```python
from build123d import *

# Parameters (mm, degrees)
F0_W         = 65
F0_H         = 45
F1_DEPTH     = 20
F2_T         = 5
F3_T1_DEPTH  = 19
F3_T3_DEPTH  = 63
F3_T5_DEPTH  = 43
F3_S9_W      = 1
F3_S9_H      = 1
F3_T10_DEPTH = 1
F3_S15_W     = 1
F3_S15_H     = 1
F3_T16_DEPTH = 1
F3_S21_W     = 1
F3_S21_H     = 1
F3_T22_DEPTH = 1
F3_S27_W     = 1
F3_S27_H     = 1
F3_T28_DEPTH = 1


# Not quite as in the source:
# - a fillet or chamfer that OpenCascade refuses, or shapes differently, is made with other operations: its cross-section is extruded or revolved along the edge and cut away or added


with BuildPart() as f1:
    # F0 (on Top) → F1 (new body)
    with BuildSketch(Plane.XY):
        Rectangle(F0_W, F0_H)
    extrude(amount=F1_DEPTH)

    # F2
    f2_openings = [f1.faces().sort_by_distance(p)[0] for p in [
        (0, 0, 20),
    ]]
    offset(amount=F2_T, openings=f2_openings, kind=Kind.INTERSECTION)

    # F3: fillet of radius 1 on 8 edges, made by hand

    # F3_s2 → F3_t1 (join)
    with BuildSketch(Plane.XY.offset(1)):
        with BuildLine():
            ThreePointArc((31.5, 22.5), (32.2071067812, 22.2071067812), (32.5, 21.5))
            Line((32.5, 21.5), (32.5, 22.5))
            Line((32.5, 22.5), (31.5, 22.5))
        make_face()
        with BuildLine():
            ThreePointArc((-31.5, 22.5), (-32.2071067812, 22.2071067812), (-32.5, 21.5))
            Line((-32.5, 21.5), (-32.5, 22.5))
            Line((-32.5, 22.5), (-31.5, 22.5))
        make_face()
        with BuildLine():
            ThreePointArc((-32.5, -21.5), (-32.2071067812, -22.2071067812), (-31.5, -22.5))
            Line((-31.5, -22.5), (-32.5, -22.5))
            Line((-32.5, -22.5), (-32.5, -21.5))
        make_face()
        with BuildLine():
            ThreePointArc((31.5, -22.5), (32.2071067812, -22.2071067812), (32.5, -21.5))
            Line((32.5, -21.5), (32.5, -22.5))
            Line((32.5, -22.5), (31.5, -22.5))
        make_face()
    extrude(amount=F3_T1_DEPTH)

    # F3_s4 → F3_t3 (join)
    with BuildSketch(Plane.YZ.offset(-31.5)):
        with BuildLine():
            ThreePointArc((22.5, 1), (22.2071067812, 0.2928932188), (21.5, 0))
            Line((21.5, 0), (22.5, 0))
            Line((22.5, 0), (22.5, 1))
        make_face()
        with BuildLine():
            ThreePointArc((-22.5, 1), (-22.2071067812, 0.2928932188), (-21.5, 0))
            Line((-21.5, 0), (-22.5, 0))
            Line((-22.5, 0), (-22.5, 1))
        make_face()
    extrude(amount=F3_T3_DEPTH)

    # F3_s6 → F3_t5 (join)
    with BuildSketch(Plane.XZ.offset(-21.5)):
        with BuildLine():
            ThreePointArc((-32.5, 1), (-32.2071067812, 0.2928932188), (-31.5, 0))
            Line((-31.5, 0), (-32.5, 0))
            Line((-32.5, 0), (-32.5, 1))
        make_face()
        with BuildLine():
            ThreePointArc((32.5, 1), (32.2071067812, 0.2928932188), (31.5, 0))
            Line((31.5, 0), (32.5, 0))
            Line((32.5, 0), (32.5, 1))
        make_face()
    extrude(amount=F3_T5_DEPTH)


with BuildPart() as f3_tool8:
    # F3_s9 → F3_t10 (new body)
    with BuildSketch(Plane.XZ.offset(-21.5)):
        with Locations((32, 0.5)):
            Rectangle(F3_S9_W, F3_S9_H)
    extrude(amount=-F3_T10_DEPTH)

    # F3_s11 → F3_t12 (revolve, cut)
    with BuildSketch(Plane(origin=(31.5, 21.5, 1), x_dir=(-0.7071067812, 0, 0.7071067812), z_dir=(-0.7071067812, 0, -0.7071067812))):
        with BuildLine():
            ThreePointArc((0, -1), (1, 0), (0, 1))
            Line((0, 1), (0, -1))
        make_face()
    revolve(axis=Axis((31.5, 21.5, 1), (0, 1, 0)), mode=Mode.SUBTRACT)


with BuildPart() as f1_1:
    add(f1.part)

    # F3_t7: union F3_tool8
    add(f3_tool8.part)


with BuildPart() as f3_tool14:
    # F3_s15 → F3_t16 (new body)
    with BuildSketch(Plane.XZ.offset(-21.5)):
        with Locations((-32, 0.5)):
            Rectangle(F3_S15_W, F3_S15_H)
    extrude(amount=-F3_T16_DEPTH)

    # F3_s17 → F3_t18 (revolve, cut)
    with BuildSketch(Plane(origin=(-31.5, 21.5, 1), x_dir=(0.7071067812, 0, 0.7071067812), z_dir=(-0.7071067812, 0, 0.7071067812))):
        with BuildLine():
            ThreePointArc((0, -1), (1, 0), (0, 1))
            Line((0, 1), (0, -1))
        make_face()
    revolve(axis=Axis((-31.5, 21.5, 1), (0, 1, 0)), mode=Mode.SUBTRACT)


with BuildPart() as f1_2:
    add(f1_1.part)

    # F3_t13: union F3_tool14
    add(f3_tool14.part)


with BuildPart() as f3_tool20:
    # F3_s21 → F3_t22 (new body)
    with BuildSketch(Plane.YZ.offset(-31.5)):
        with Locations((-22, 0.5)):
            Rectangle(F3_S21_W, F3_S21_H)
    extrude(amount=-F3_T22_DEPTH)

    # F3_s23 → F3_t24 (revolve, cut)
    with BuildSketch(Plane(origin=(-31.5, -21.5, 1), x_dir=(0, 0.7071067812, 0.7071067812), z_dir=(0, -0.7071067812, 0.7071067812))):
        with BuildLine():
            ThreePointArc((0, -1), (1, 0), (0, 1))
            Line((0, 1), (0, -1))
        make_face()
    revolve(axis=Axis((-31.5, -21.5, 1), (-1, 0, 0)), mode=Mode.SUBTRACT)


with BuildPart() as f1_3:
    add(f1_2.part)

    # F3_t19: union F3_tool20
    add(f3_tool20.part)


with BuildPart() as f3_tool26:
    # F3_s27 → F3_t28 (new body)
    with BuildSketch(Plane.XZ.offset(21.5)):
        with Locations((32, 0.5)):
            Rectangle(F3_S27_W, F3_S27_H)
    extrude(amount=F3_T28_DEPTH)

    # F3_s29 → F3_t30 (revolve, cut)
    with BuildSketch(Plane(origin=(31.5, -21.5, 1), x_dir=(-0.7071067812, 0, 0.7071067812), z_dir=(0.7071067812, 0, 0.7071067812))):
        with BuildLine():
            ThreePointArc((0, -1), (1, 0), (0, 1))
            Line((0, 1), (0, -1))
        make_face()
    revolve(axis=Axis((31.5, -21.5, 1), (0, -1, 0)), mode=Mode.SUBTRACT)


with BuildPart() as f1_4:
    add(f1_3.part)

    # F3_t25: union F3_tool26
    add(f3_tool26.part)


solid = f1_4.part
```
Model file for the job. Use its own axes, mm. A direction names the side the tool comes from. Coordinates: 2 decimals unless noted, no trailing zeros. Write each loop counter-clockwise with the first axis right and the second up, starting at its lowest first coordinate (ties: lowest second). Pieces come first, ordered by that corner, then holes. Notation, with made-up numbers: (67.5, 77.25) - (125.5, 77.25) arc R20 ccw to (125.5, 91.25) - close; hole circle Ø2 at (74, 24). An arc over 180 degrees is marked (long way). One line per item, written item: value. Start each with the question number.
1. Flat gauge pin, fed straight in: pin 1 (13 mm diameter, centred on x = -2.5, y = 3, fed in from +Z). Where does the tip first touch, or does it go through?
2. Mould opens along X. For faces 3 (the flat face through (32.5, 0, 10)), 4 (the flat face through (-37.5, 0, 7)), 5 (the flat face through (-1, -27.5, 7)) say: released by +X, released by -X, zero draft, split by the parting line, or undercut.
3. Tool access for faces 1 (the flat face through (-32.5, 0, 10)), 2 (the flat face through (-1, 0, -5)): list every direction of +Z, -Z, +X, -X, +Y, -Y with a clear straight run to the whole face (end or side of a thin tool).
4. Slice it at A-A (z = 10.5). Write the cut outline in (x, y).
5. Slice it at C-C (x = -4.5). Write the cut outline in (y, z).
6. Slice it at B-B (y = -1.5). Write the cut outline in (x, z), plus the area to 3 significant figures.
7. Probe line 1 (X direction, y = 11.5, z = 7); line 2 (Y direction, x = -9, z = 4.5); line 3 (Z direction, x = 11, y = -17). List the from-to ranges inside material, lowest first. Write a range as from..to.
Answers below:
1. pin 1: stops at z = 0
2. face 3: undercut
2. face 4: released by -X
2. face 5: zero draft
3. face 1: +Z
3. face 2: -Z, +X, -X, +Y, -Y
4. outline: (-37.5, -27.5) - (37.5, -27.5) - (37.5, 27.5) - (-37.5, 27.5) - close; hole (-32.5, -21.5) arc R1 ccw to (-31.5, -22.5) - (31.5, -22.5) arc R1 ccw to (32.5, -21.5) - (32.5, 21.5) arc R1 ccw to (31.5, 22.5) - (-31.5, 22.5) arc R1 ccw to (-32.5, 21.5) - close
5. outline: (-27.5, -5) - (27.5, -5) - (27.5, 20) - (22.5, 20) - (22.5, 1) arc R1 cw to (21.5, 0) - (-21.5, 0) arc R1 cw to (-22.5, 1) - (-22.5, 20) - (-27.5, 20) - close
6. outline: (-37.5, -5) - (37.5, -5) - (37.5, 20) - (32.5, 20) - (32.5, 1) arc R1 cw to (31.5, 0) - (-31.5, 0) arc R1 cw to (-32.5, 1) - (-32.5, 20) - (-37.5, 20) - close
6. area: 575 mm^2
7. line 1: x = -37.5..-32.5, 32.5..37.5
7. line 2: y = -27.5..-22.5, 22.5..27.5
7. line 3: z = -5..0
